```python
from build123d import *

# Parameters (mm, degrees)
F_8_1_8_1_DURCHMESSER_BOHRUNG1_D = 8.1
SKIZZE4_R                        = 1.25
SCHNITT_LINEAR_AUSTRAGEN1_DEPTH  = 47.652974182
SKIZZE5_R                        = 1.55
SCHNITT_LINEAR_AUSTRAGEN2_DEPTH  = 47.652974182
FASE2_SIZE                       = 3.5


with BuildPart() as part:
    # Skizze1 → Rotation1 (revolve)
    with BuildSketch(Plane.XY, mode=Mode.PRIVATE) as rotation1_sk:
        Polygon((0, 0), (0, 16.5), (3, 16.5), (3, 32.5), (8, 32.5), (8, 0), align=None)
    revolve(rotation1_sk.sketch.rotate(Axis((0, 0, 0), (-1, 0, 0)), 90), axis=Axis((0, 0, 0), (-1, 0, 0)))

    # Ø8.1 (8.1) Durchmesser Bohrung1 (through all)
    with Locations(Plane.ZY):
        with Locations((0, 0)):
            Hole(F_8_1_8_1_DURCHMESSER_BOHRUNG1_D / 2)

    # Skizze4 → Schnitt-Linear austragen1 (cut, through all)
    with BuildSketch(Plane(origin=(8, 0, 0), x_dir=(0, 0, -1), z_dir=(1, 0, 0))):
        with Locations((0, 10)):
            Circle(SKIZZE4_R)
        with Locations((8.660254038, -5)):
            Circle(SKIZZE4_R)
        with Locations((-8.660254038, -5)):
            Circle(SKIZZE4_R)
    extrude(amount=-SCHNITT_LINEAR_AUSTRAGEN1_DEPTH, mode=Mode.SUBTRACT)

    # Skizze5 → Schnitt-Linear austragen2 (cut, through all)
    with BuildSketch(Plane(origin=(8, 0, 0), x_dir=(0, 0, -1), z_dir=(1, 0, 0))):
        with Locations((0, 25)):
            Circle(SKIZZE5_R)
        with Locations((21.650635095, 12.5)):
            Circle(SKIZZE5_R)
        with Locations((21.650635095, -12.5)):
            Circle(SKIZZE5_R)
        with Locations((0, -25)):
            Circle(SKIZZE5_R)
        with Locations((-21.650635095, -12.5)):
            Circle(SKIZZE5_R)
        with Locations((-21.650635095, 12.5)):
            Circle(SKIZZE5_R)
    extrude(amount=-SCHNITT_LINEAR_AUSTRAGEN2_DEPTH, mode=Mode.SUBTRACT)

    # Fase2
    fase2_edges = [part.edges().sort_by_distance(p)[0] for p in [
        (3, 25, 1.55),
        (3, 12.5, 23.200635095),
        (3, -12.5, 23.200635095),
        (3, -25, 1.55),
        (3, -12.5, -20.100635095),
        (3, 12.5, -20.100635095),
    ]]
    chamfer(fase2_edges, length=FASE2_SIZE)


solid = part.part
```
Here's how the part is built. I have some questions about the finished solid (model axes, mm). Give positions to 0.01 mm unless a question says otherwise; leave off trailing zeros. Write each loop counter-clockwise with the first axis right and the second up, starting at its lowest first coordinate (ties: lowest second). Pieces come first, ordered by that corner, then holes.
(1) Imagine slicing it at B-B, the plane x = 7.25. Count the separate pieces of the cut face and the enclosed holes in it, and give its area (3 significant figures).
Output values:
separate pieces: 1
enclosed holes: 10
area: 3,210 mm2
(2) Imagine slicing it at C-C, the plane y = -5. Write out the boundary of the cut face in (x, z), and give its area (3 significant figures).
Output values:
outline: (0, -15.72) - (3, -15.72) - (3, -32.11) - (8, -32.11) - (8, -9.91) - (0, -9.91) - close; (0, -7.41) - (8, -7.41) - (8, 7.41) - (0, 7.41) - close; (0, 9.91) - (8, 9.91) - (8, 32.11) - (3, 32.11) - (3, 15.72) - (0, 15.72) - close
area: 375 mm2
(3) Will these pins go through, and if not, where does the flat tip stop? pin 1 (4 mm diameter, centred on y = -12.5, z = -21.65, fed in from -X); pin 2 (2 mm diameter, centred on x = 7, y = -16, fed in from +Z); pin 3 (1.5 mm diameter, centred on y = 10, z = 0, fed in from -X); pin 4 (1 mm diameter, centred on x = 7, y = 15.5, fed in from -Z).
Output values:
pin 1: stops at x = 6.05
pin 2: stops at z = 28.83
pin 3: passes through
pin 4: stops at z = -28.83
(4) Imagine slicing it at D-D, the plane y = -25. Write out the boundary of the cut face in (x, z).
Output values:
outline: (3, -20.77) - (8, -20.77) - (8, -1.55) - (6.5, -1.55) - (3, -5.05) - close; (3, 5.05) - (6.5, 1.55) - (8, 1.55) - (8, 20.77) - (3, 20.77) - close
(5) Imagine slicing it at A-A, the plane x = 1.5. Write out the boundary of the cut face in (y, z), and give its area (3 significant figures).
Output values:
outline: circle Ø33 at (0, 0); hole circle Ø2.5 at (-5, -8.66); hole circle Ø2.5 at (-5, 8.66); hole circle Ø8.1 at (0, 0); hole circle Ø2.5 at (10, 0)
area: 789 mm2
(6) If I drill on L1, parallel to Y at x = 7, z = 0; L2, parallel to Y at x = 2, z = 0; L3, parallel to Z at x = 5.5, y = 12.5, over which ranges is the centre line in solid material (lowest first)?
Output values:
L1: y = -32.5 to -26.55, -23.45 to -4.05, 4.05 to 8.75, 11.25 to 23.45, 26.55 to 32.5
L2: y = -16.5 to -4.05, 4.05 to 8.75, 11.25 to 16.5
L3: z = -30 to -24.2, -19.1 to 19.1, 24.2 to 30
(7) Thinking about a two-plate mould opening in Z: for faces 1 (the face through (8, 0, -7)), 2 (the face through (4.06, 11.24, 0.16)), 3 (the face through (1.521, -4.956, -15.738)), which applies, pulls with the +Z half, pulls with the -Z half, needs draft (parallel to the pull), parting line crosses it, or undercut?
Output values:
face 1: needs draft
face 2: undercut
face 3: parting line crosses it
